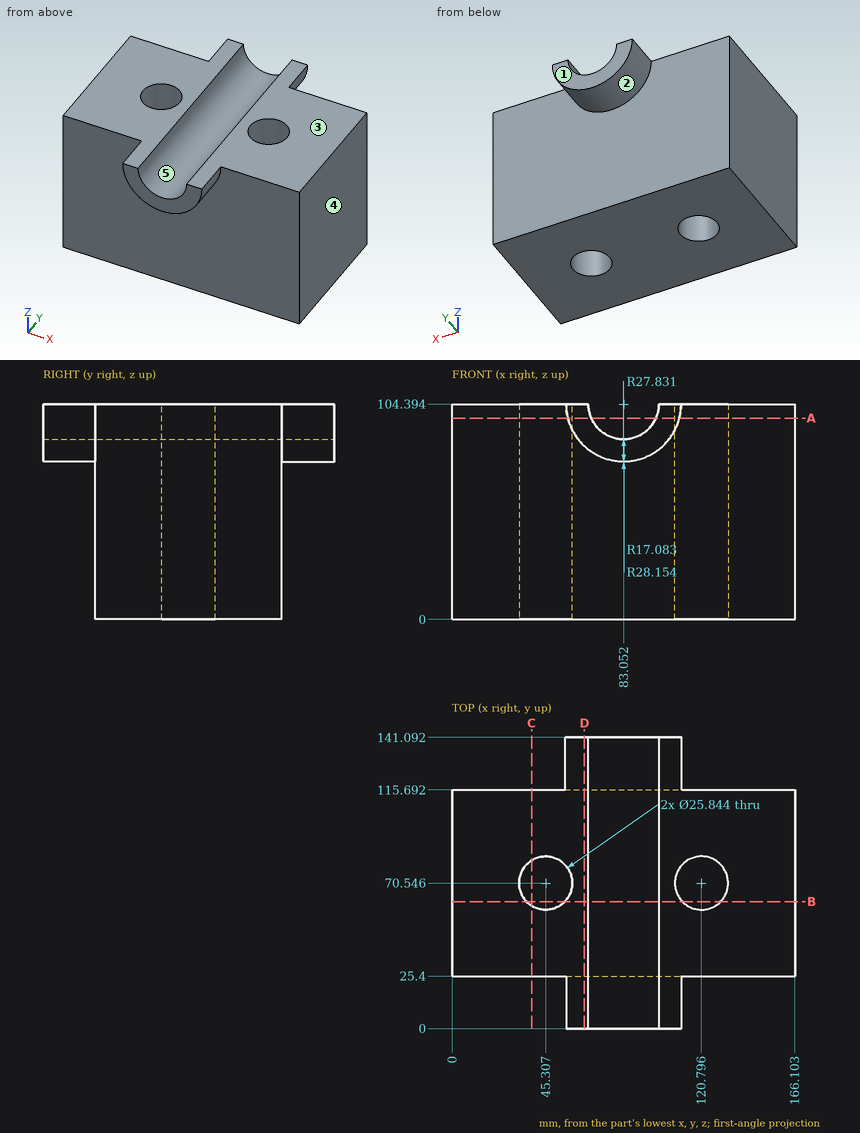
Here's the drawing with two shaded views (mm, measured from the low corner). I have some questions. A direction names the side the tool comes from. Give positions to 0.01 mm unless a question says otherwise; leave off trailing zeros. Order: outer loops, then holes, each group sorted by start corner. A loop starts at its lowest first (then second) coordinate and runs counter-clockwise, first axis right, second up. Notation, with made-up numbers: M 18,57 L 47,57 A34 ccw 47,89 Z; hole C 75,33.5 d1. An arc over 180 degrees is marked long. Answer as a JSON object with one key per item and string values. Group by question number.
1) I'm going to push flat-ended pins straight in: pin 1 Ø3 at (x, z) = (111, 67) entering from +Y; pin 2 Ø20.5 at (x, y) = (120.8, 70.55) entering from +Z. Where does each tip first touch, or does it pass through?
2) We'd pull the mould along X, two halves only. Please class the marked faces 3, 4 and 5: pulls with the +X half, pulls with the -X half, needs draft (parallel to the pull), parting line crosses it, or undercut.
3) Suppose I cut it at B-B, the plane y = 61.5. Write out the boundary of the cut face in (x, z) (1 decimal).
4) Suppose I cut it at D-D, the plane x = 64. Write out the boundary of the cut face in (y, z) (1 decimal).
5) Suppose I cut it at A-A, the plane z = 97.5. Write out the boundary of the cut face in (x, y) (1 decimal).
6) On a 3-axis mill with a long thin cutter (end or side, diameter ignored), from which of +Z, -Z, +X, -X, +Y, -Y can I reach the whole of each face in a straight line? I mean the marked faces 1 and 2. Say none if no direction works.
7) Please list where these lines run through material, in increasing order: L1, parallel to X at y = 70, z = 34.5; L2, parallel to Y at x = 45.5, z = 12.5 (1 decimal); L3, parallel to X at y = 81, z = 26.5 (1 decimal). Write a range as [from, to].
8) Suppose I cut it at C-C, the plane x = 38.5. Write out the boundary of the cut face in (y, z) (1 decimal), plus the area to 3 significant figures.
Results found:
{
 "1": {"pin 1": "y = 115.69", "pin 2": "through"},
 "2": {"face 3": "needs draft", "face 4": "pulls with the +X half", "face 5": "undercut"},
 "3": {"outline": "M 0,0 L 36.1,0 L 36.1,104.4 L 0,104.4 Z; M 54.5,0 L 111.6,0 L 111.6,104.4 L 100.1,104.4 A17.1 cw 66,104.4 L 54.5,104.4 Z; M 130,0 L 166.1,0 L 166.1,104.4 L 130,104.4 Z"},
 "4": {"outline": "M 0,84.1 L 25.4,84.1 L 25.4,0 L 115.7,0 L 115.7,83.7 L 141.1,83.7 L 141.1,104.4 L 0,104.4 Z"},
 "5": {"outline": "M 0,25.4 L 56.1,25.4 L 56.1,0 L 67.4,0 L 67.4,141.1 L 55.8,141.1 L 55.8,115.7 L 0,115.7 Z; M 98.7,0 L 110,0 L 110,25.4 L 166.1,25.4 L 166.1,115.7 L 110.3,115.7 L 110.3,141.1 L 98.7,141.1 Z; hole C 45.3,70.5 d25.8; hole C 120.8,70.5 d25.8"},
 "6": {"face 1": "+Z, -Z, +X, -X, +Y", "face 2": "-Z, +Y"},
 "7": {"L1": "[0, 32.4], [58.22, 107.89], [133.71, 166.1]", "L2": "[25.4, 57.6], [83.5, 115.7]", "L3": "[0, 37.7], [52.9, 113.2], [128.4, 166.1]"},
 "8": {"outline": "M 25.4,0 L 59.6,0 L 59.6,104.4 L 25.4,104.4 Z; M 81.5,0 L 115.7,0 L 115.7,104.4 L 81.5,104.4 Z", "area": "7,130 mm²"}
}
